Autodesk Fusion 360 part; units mm, degrees
sketch "Sketch1" plane through (0, 0, 0) normal (1, 0, 0) x (0, 1, 0)
  line L0 (0, 0) -> (2.54, 0)
  line L1 (2.54, 0) -> (2.54, 50.8)
  line L2 (2.54, 50.8) -> (0, 50.8)
  line L3 (0, 50.8) -> (0, 0)
  line L4 (0, 50.8) -> (53.34, 50.8)
  line L5 (53.34, 50.8) -> (53.34, 48.26)
  line L6 (53.34, 48.26) -> (0, 48.26)
  line L7 (0, 48.26) -> (0, 50.8)
  dimension "d5" = 2.54
  dimension "d6" = 50.8
  dimension "d7" = 53.34
  dimension "d8" = 2.54
extrude "Extrude1" add sketch "Sketch1" along normal blind 50.8 contours L1 L4 L5 L6
extrude "Extrude2" add sketch "Sketch1" along normal blind 50.8 contours L1 L2 L3 L4 L6 L7
extrude "Extrude3" add sketch "Sketch1" along normal blind 50.8 contours L0 L1 L3 L6
sketch "Sketch3" plane through (0, 0, 50.8) normal (0, 0, 1) x (-1, 0, 0)
  line L0 (0, -53.34) -> (0, 0)
  line L1 (0, 0) -> (-50.8, 0)
  line L2 (-50.8, 0) -> (-50.8, -53.34)
  line L3 (-50.8, -53.34) -> (0, -53.34)
  circle A0 centre (-15.24, -43.18) radius 2.3813
  circle A1 centre (-32.7025, -43.18) radius 2.3813
  circle A2 centre (-15.24, -25.7175) radius 2.3813
  circle A3 centre (-32.7025, -25.7175) radius 2.3813
  dimension "d15" = 17.4625
  dimension "d16" = 17.4625
  dimension "d17" = 4.7625
  dimension "d18" = 4.7625
  dimension "d19" = 4.7625
  dimension "d20" = 4.7625
hole "Hole1" at (32.7025, 43.18, 50.8) direction (0, 0, -1) diameter 4.7625 depth 22.86 tip angle 118
hole "Hole2" at (15.24, 43.18, 50.8) at (15.24, 25.7175, 50.8) at (32.7025, 25.7175, 50.8) direction (0, 0, -1) diameter 4.7752 depth 22.86 tip angle 118
sketch "Sketch4" plane through (0, 0, 0) normal (0, -1, 0) x (1, 0, 0)
  line L0 (0, 50.8) -> (0, 0)
  line L1 (0, 0) -> (50.8, 0)
  line L2 (50.8, 0) -> (50.8, 50.8)
  line L3 (50.8, 50.8) -> (0, 50.8)
  line L4 (0, 50.8) -> (15.2337, 50.8)
  line L5 (15.2337, 50.8) -> (15.2337, 40.6463)
  line L6 (15.2337, 40.6463) -> (32.6962, 40.6463)
  line L7 (32.6962, 40.6463) -> (32.6962, 23.1838)
  line L8 (32.6962, 23.1838) -> (15.2337, 23.1838)
  line L9 (15.2337, 23.1838) -> (15.2337, 40.6463)
  circle A0 centre (15.2337, 40.6463) radius 2.3812
  circle A1 centre (32.6962, 40.6463) radius 2.3812
  circle A2 centre (15.2337, 23.1838) radius 2.3813
  circle A3 centre (32.6962, 23.1838) radius 2.3812
  dimension "d42" = 15.2336
  dimension "d43" = 10.1537
  dimension "d44" = 17.4625
  dimension "d45" = 17.4625
  dimension "d46" = 4.7625
  dimension "d47" = 4.7625
  dimension "d48" = 4.7625
  dimension "d49" = 4.7625
hole "Hole3" at (15.2337, 0, 40.6463) at (15.2337, 0, 23.1838) at (32.6962, 0, 40.6463) at (32.6962, 0, 23.1838) direction (0, 1, 0) diameter 4.7752 depth 22.86 tip angle 118
sketch "Sketch6" plane through (50.8, 0, 0) normal (1, 0, 0) x (0, 1, 0)
  line L0 (53.34, 48.26) -> (53.34, 50.8)
  line L1 (53.34, 50.8) -> (0, 50.8)
  line L2 (0, 50.8) -> (0, 0)
  line L3 (0, 0) -> (2.54, 0)
  line L4 (2.54, 0) -> (2.54, 48.26)
  line L5 (2.54, 48.26) -> (53.34, 48.26)
equation "d15 = ( 11 / 16 ) * 1 in"
equation "d16 = ( 11 / 16 ) * 1 in"
equation "d17 = ( 3 / 16 ) * 1 in"
equation "d18 = ( 3 / 16 ) * 1 in"
equation "d19 = ( 3 / 16 ) * 1 in"
equation "d20 = ( 3 / 16 ) * 1 in"
equation "d42 = 0.506 in + ( 3 / 32 ) * 1 in"
equation "d43 = 0.306 in + ( 3 / 32 ) * 1 in"
equation "d44 = ( 11 / 16 ) * 1 in"
equation "d45 = ( 11 / 16 ) * 1 in"
equation "d46 = ( 3 / 16 ) * 1 in"
equation "d47 = ( 3 / 16 ) * 1 in"
equation "d48 = ( 3 / 16 ) * 1 in"
equation "d49 = ( 3 / 16 ) * 1 in"
Check sheet for the modelled part. Datum: model origin and axes. Units: mm. A direction names the side the tool comes from. Coordinates: 2 decimals unless noted, no trailing zeros. Order: outer loops, then holes, each group sorted by start corner. A loop starts at its lowest first (then second) coordinate and runs counter-clockwise, first axis right, second up. Notation, with made-up numbers: M 65,-3.5 L 124,-3.5 A28 ccw 124,28.5 Z; hole C 15.25,-12.75 d9. An arc over 180 degrees is marked long. Write each question's results on one line, items separated by ' | '. Start each with the question number.
1. Mould release check, pull along Y, two halves, no side actions. Record for faces 1 (the face through (14.52, 23.44, 49.51)), 2 (the face through (25, 28, 48.26)), 3 (the face through (30.69, 24.43, 49.51)), 4 (the face through (25, 53.34, 50)): +Y half, -Y half, draft (parallel to the pull), parting line (faces both ways), or undercut.
2. Go/stop test with flat-tipped pins: P1, Ø24, axis at x = 32.5, z = 33.5, coming from the +Y side; P2, Ø1, axis at x = 28, y = 44.5, coming from the -Z side. Record where each tip stops, or that it passes through.
3. Access from +Z, -Z, +X, -X, +Y, -Y to the whole of each face (thin tool, end or side, straight path). Record for faces 5 (the face through (14.523, 40.903, 49.512)), 6 (the face through (25, 2.54, 24)).
4. Material ranges on probe 1 along X at (y, z) = (43.18, 49); probe 2 along Y at (x, z) = (15, 49); probe 3 along Y at (x, z) = (13.5, 10.5), recorded low to high.
5. Cross-section at A-A on y = 43.18. Record the cut outline in (x, z).
6. Cross-section at B-B on x = 41. Record the cut outline in (y, z).
7. Cross-section at C-C on z = 10. Record the cut outline in (x, y).
Checks:
1) face 1: undercut | face 2: draft | face 3: undercut | face 4: +Y half
2) P1: stops at y = 2.54 | P2: stops at z = 48.26
3) face 5: +Z, -Z | face 6: -Z, +X, -X, +Y
4) probe 1: x = 0 to 12.85, 17.63 to 30.32, 35.08 to 50.8 | probe 2: y = 0 to 23.34, 28.09 to 40.8, 45.56 to 53.34 | probe 3: y = 0 to 2.54
5) outline: M 0,48.26 L 12.85,48.26 L 12.85,50.8 L 0,50.8 Z; M 17.63,48.26 L 30.32,48.26 L 30.32,50.8 L 17.63,50.8 Z; M 35.08,48.26 L 50.8,48.26 L 50.8,50.8 L 35.08,50.8 Z
6) outline: M 0,0 L 2.54,0 L 2.54,48.26 L 53.34,48.26 L 53.34,50.8 L 0,50.8 Z
7) outline: M 0,0 L 50.8,0 L 50.8,2.54 L 0,2.54 Z
